Input: part model. Units: mm. Frame: model coordinates. A direction names the side the tool comes from. Give positions to 0.01 mm unless a question says otherwise; leave off trailing zeros. Loops run counter-clockwise (first coordinate to the right, second up) from the corner with the lowest first, then second, coordinate; pieces in that order, holes last. Notation, with made-up numbers: (62.25, -21.5) -> (81.25, -21.5) arc R25 cw to (81.25, 0.5) -> close; hole circle Ø7 at (60, 63.25). An arc over 180 degrees is marked (long way). Answer in a Markdown table with one row per item. Add a question column.
```python
from build123d import *

# Parameters (mm, degrees)
F0_R     = 11.05
F1_DEPTH = 7
F2_R     = 2


with BuildPart() as f1:
    # F0 (on Top) → F1 (new body)
    with BuildSketch(Plane.XY):
        with BuildLine():
            Line((-10.1438404956, 11.05), (0, 11.05))
            Line((0, 11.05), (10.1438404956, 11.05))
            ThreePointArc((10.1438404956, 11.05), (5.4428852643, 13.9776607485), (0, 15))
            ThreePointArc((0, 15), (-5.4428852643, 13.9776607485), (-10.1438404956, 11.05))
        make_face()
        with BuildLine():
            Line((10.1438404956, -11.05), (0, -11.05))
            Line((0, -11.05), (-10.1438404956, -11.05))
            ThreePointArc((-10.1438404956, -11.05), (-5.442885249, -13.9776607544), (3.27e-08, -15))
            ThreePointArc((3.27e-08, -15), (5.4428852795, -13.9776607426), (10.1438404956, -11.05))
        make_face()
        with BuildLine():
            Line((-17.8561595044, 11.05), (-10.1438404956, 11.05))
            ThreePointArc((-10.1438404956, 11.05), (-5.4428852643, 13.9776607485), (0, 15))
            Line((0, 15), (-28, 15))
            ThreePointArc((-28, 15), (-22.5571147357, 13.9776607485), (-17.8561595044, 11.05))
        make_face()
        with BuildLine():
            ThreePointArc((0, 15), (5.4428852643, 13.9776607485), (10.1438404956, 11.05))
            Line((10.1438404956, 11.05), (17.8561595044, 11.05))
            ThreePointArc((17.8561595044, 11.05), (22.5571147357, 13.9776607485), (28, 15))
            Line((28, 15), (0, 15))
        make_face()
        with BuildLine():
            ThreePointArc((3.27e-08, -15), (-5.442885249, -13.9776607544), (-10.1438404956, -11.05))
            Line((-10.1438404956, -11.05), (-17.8561595044, -11.05))
            ThreePointArc((-17.8561595044, -11.05), (-22.5571147357, -13.9776607485), (-28, -15))
            Line((-28, -15), (3.27e-08, -15))
        make_face()
        with BuildLine():
            Line((17.8561595044, -11.05), (10.1438404956, -11.05))
            ThreePointArc((10.1438404956, -11.05), (5.4428852795, -13.9776607426), (3.27e-08, -15))
            Line((3.27e-08, -15), (28, -15))
            ThreePointArc((28, -15), (22.5571147357, -13.9776607485), (17.8561595044, -11.05))
        make_face()
        with BuildLine():
            ThreePointArc((-14, -5.3851648071), (-15, 0), (-14, 5.3851648071))
            ThreePointArc((-14, 5.3851648071), (-15.6002480706, 8.4407435745), (-17.8561595044, 11.05))
            ThreePointArc((-17.8561595044, 11.05), (-22.5571147357, 13.9776607485), (-28, 15))
            ThreePointArc((-28, 15), (-43, 0), (-28, -15))
            ThreePointArc((-28, -15), (-22.5571147357, -13.9776607485), (-17.8561595044, -11.05))
            ThreePointArc((-17.8561595044, -11.05), (-15.6002480706, -8.4407435745), (-14, -5.3851648071))
        make_face()
        with Locations((-28, 0)):
            Circle(F0_R, mode=Mode.SUBTRACT)
        with BuildLine():
            ThreePointArc((17.8561595044, 11.05), (15.6002480706, 8.4407435745), (14, 5.3851648071))
            ThreePointArc((14, 5.3851648071), (14.7478812038, 2.7386127875), (15, 0))
            ThreePointArc((15, 0), (14.7478812038, -2.7386127875), (14, -5.3851648071))
            ThreePointArc((14, -5.3851648071), (15.6002480706, -8.4407435745), (17.8561595044, -11.05))
            ThreePointArc((17.8561595044, -11.05), (22.5571147357, -13.9776607485), (28, -15))
            ThreePointArc((28, -15), (38.6066017178, -10.6066017178), (43, 0))
            ThreePointArc((43, 0), (38.6066017178, 10.6066017178), (28, 15))
            ThreePointArc((28, 15), (22.5571147357, 13.9776607485), (17.8561595044, 11.05))
        make_face()
        with Locations((28, 0)):
            Circle(F0_R, mode=Mode.SUBTRACT)
        with BuildLine():
            ThreePointArc((-13, 0), (-13.2521187962, 2.7386127875), (-14, 5.3851648071))
            ThreePointArc((-14, 5.3851648071), (-15, 0), (-14, -5.3851648071))
            ThreePointArc((-14, -5.3851648071), (-13.2521187962, -2.7386127875), (-13, 0))
        make_face()
        with BuildLine():
            ThreePointArc((0, -11.05), (-11.05, 0), (0, 11.05))
            Line((0, 11.05), (-10.1438404956, 11.05))
            ThreePointArc((-10.1438404956, 11.05), (-12.3997519294, 8.4407435745), (-14, 5.3851648071))
            ThreePointArc((-14, 5.3851648071), (-13.2521187962, 2.7386127875), (-13, 0))
            ThreePointArc((-13, 0), (-13.2521187962, -2.7386127875), (-14, -5.3851648071))
            ThreePointArc((-14, -5.3851648071), (-12.3997519294, -8.4407435745), (-10.1438404956, -11.05))
            Line((-10.1438404956, -11.05), (0, -11.05))
        make_face()
        with BuildLine():
            ThreePointArc((0, 11.05), (7.8135299321, 7.8135299321), (11.05, 0))
            ThreePointArc((11.05, 0), (7.8135299321, -7.8135299321), (0, -11.05))
            Line((0, -11.05), (10.1438404956, -11.05))
            ThreePointArc((10.1438404956, -11.05), (12.3997519294, -8.4407435745), (14, -5.3851648071))
            ThreePointArc((14, -5.3851648071), (13, 0), (14, 5.3851648071))
            ThreePointArc((14, 5.3851648071), (12.3997519294, 8.4407435745), (10.1438404956, 11.05))
            Line((10.1438404956, 11.05), (0, 11.05))
        make_face()
        with BuildLine():
            ThreePointArc((15, 0), (14.7478812038, 2.7386127875), (14, 5.3851648071))
            ThreePointArc((14, 5.3851648071), (13, 0), (14, -5.3851648071))
            ThreePointArc((14, -5.3851648071), (14.7478812038, -2.7386127875), (15, 0))
        make_face()
    extrude(amount=F1_DEPTH)

    # F2
    f2_edges = [f1.edges().sort_by_distance(p)[0] for p in [
        (0, 15, 7),
        (0, -15, 0),
    ]]
    fillet(f2_edges, radius=F2_R)


solid = f1.part
```
1) Section C-C on y = 8.25. State how many separate pieces and enclosed holes the cut face has, and give its area (3 significant figures).
2) Reachability of faces 1 (the face through (14, 11.05, 3)), 2 (the face through (-10, -6, 7)) from +Z, -Z, +X, -X, +Y, -Y: full face, straight path, thin tool, end or side. Return the list, or none.
3) Section A-A on z = 3.25. Output: boundary loops of the cut face in (x, y).
4) Pin query (flat end, axial travel): pin 1 (4 mm diameter, centred on y = -11.5, z = 4, fed in from -X); pin 2 (1 mm diameter, centred on x = -29, z = 4, fed in from +Y); pin 3 (13.5 mm diameter, centred on x = -28, y = 0, fed in from +Z); pin 4 (1 mm diameter, centred on y = -1.5, z = 2, fed in from -X). Return the tip coordinate at first contact, or that it passes through.
5) Material intervals for line 1 along Y through (x, z) = (28, 3.25); line 2 along X through (y, z) = (1, 3.25); line 3 along X through (y, z) = (-2.75, 4.5), sorted ascending.
6) Pull-direction query (Y, two-part tool) for faces 3 (the face through (0, 15, 3)), 4 (the face through (0.39, -14.43, 0.6)), 5 (the face through (15.628, 8.481, 3.451)); classes: +Y half, -Y half, draft (parallel to the pull), parting line (faces both ways), or undercut.
7) Section B-B on x = -6. Output: boundary loops of the cut face in (y, z), and give its area (3 significant figures).
Working result:
| question | item | result |
|---|---|---|
| 1 | separate pieces | 6 |
| 1 | enclosed holes | 0 |
| 1 | area | 213 mm2 |
| 2 | face 1 | +Z, -Z |
| 2 | face 2 | +Z, +X, -X, +Y, -Y |
| 3 | outline | (-28, -15) -> (28, -15) arc R15 ccw to (28, 15) -> (-28, 15) arc R15 ccw to start; hole circle Ø22.1 at (-28, 0); hole (-17.86, -11.05) -> (-10.14, -11.05) arc R15 cw to (-14, -5.39) arc R15 cw to start; hole (-17.86, 11.05) arc R15 cw to (-14, 5.39) arc R15 cw to (-10.14, 11.05) -> close; hole circle Ø22.1 at (0, 0); hole (10.14, -11.05) -> (17.86, -11.05) arc R15 cw to (14, -5.39) arc R15 cw to start; hole (10.14, 11.05) arc R15 cw to (14, 5.39) arc R15 cw to (17.86, 11.05) -> close; hole circle Ø22.1 at (28, 0) |
| 4 | pin 1 | stops at x = -39.61 |
| 4 | pin 2 | stops at y = 14.99 |
| 4 | pin 3 | passes through |
| 4 | pin 4 | stops at x = -42.97 |
| 5 | line 1 | y = -15 to -11.05, 11.05 to 15 |
| 5 | line 2 | x = -42.97 to -39, -17 to -11, 11 to 17, 39 to 42.97 |
| 5 | line 3 | x = -42.75 to -38.7, -17.3 to -10.7, 10.7 to 17.3, 38.7 to 42.75 |
| 6 | face 3 | +Y half |
| 6 | face 4 | -Y half |
| 6 | face 5 | undercut |
| 7 | outline | (-15, 2) arc R2 ccw to (-13, 0) -> (-9.28, 0) -> (-9.28, 7) -> (-13, 7) arc R2 ccw to (-15, 5) -> close; (9.28, 0) -> (13, 0) arc R2 ccw to (15, 2) -> (15, 5) arc R2 ccw to (13, 7) -> (9.28, 7) -> close |
| 7 | area | 76.7 mm2 |
